The model under review builds one solid part; all positions refer to its coordinate system, in mm. Coordinates: 2 decimals unless noted, no trailing zeros. Write each loop counter-clockwise with the first axis right and the second up, starting at its lowest first coordinate (ties: lowest second). Pieces come first, ordered by that corner, then holes. Notation, with made-up numbers: (-5.5, -8) - (46.5, -8) arc R27 ccw to (46.5, 17) - close; hole circle Ø9 at (28, 17). An arc over 180 degrees is marked (long way). Answer as CSV lines item,"result". Start each with the question number.
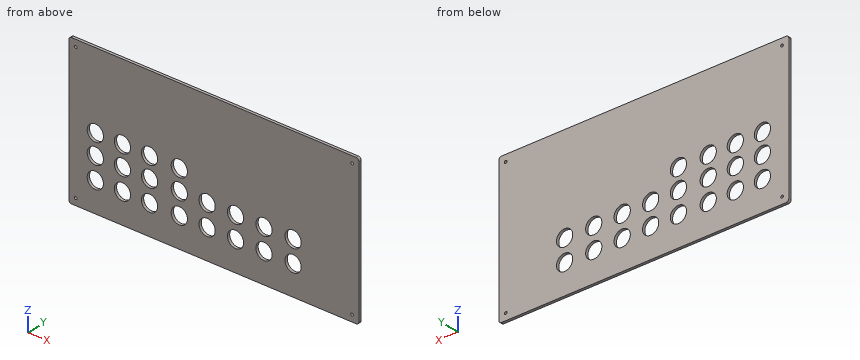
```python
from build123d import *

# Parameters (mm, degrees)
BOSS_EXTRUDE1_DEPTH       = 2
SKETCH3_R                 = 6
CUT_EXTRUDE1_DEPTH        = 3
F_2_0MM_DOWEL_HOLE1_D     = 2
F_2_0MM_DOWEL_HOLE1_DEPTH = 8
F_2_0MM_DOWEL_HOLE1_TIP   = 0.600860619


with BuildPart() as part:
    # Sketch2 → Boss-Extrude1 (new body)
    with BuildSketch(Plane(origin=(0, 0, 0), x_dir=(1, 0, 0), z_dir=(0, 1, 0))):
        with BuildLine():
            Line((105, 54.5), (-105, 54.5))
            ThreePointArc((-105, 54.5), (-106.414213562, 53.914213562), (-107, 52.5))
            Line((-107, 52.5), (-107, -52.5))
            ThreePointArc((-107, -52.5), (-106.414213562, -53.914213562), (-105, -54.5))
            Line((-105, -54.5), (105, -54.5))
            ThreePointArc((105, -54.5), (106.414213562, -53.914213562), (107, -52.5))
            Line((107, -52.5), (107, 52.5))
            ThreePointArc((107, 52.5), (106.414213562, 53.914213562), (105, 54.5))
        make_face()
    extrude(amount=BOSS_EXTRUDE1_DEPTH)

    # Sketch3 → Cut-Extrude1 (cut)
    with BuildSketch(Plane(origin=(0, 2, 0), x_dir=(1, 0, 0), z_dir=(0, 1, 0))):
        with Locations((-87.5, 32.5)):
            Circle(SKETCH3_R)
        with Locations((-67.5, 32.5)):
            Circle(SKETCH3_R)
        with Locations((-47.5, 32.5)):
            Circle(SKETCH3_R)
        with Locations((-25.5, 32.5)):
            Circle(SKETCH3_R)
        with Locations((-5, 32.5)):
            Circle(SKETCH3_R)
        with Locations((16, 32.5)):
            Circle(SKETCH3_R)
        with Locations((37, 32.5)):
            Circle(SKETCH3_R)
        with Locations((58.5, 32.5)):
            Circle(SKETCH3_R)
        with Locations((-87.5, 16.5)):
            Circle(SKETCH3_R)
        with Locations((-67.5, 16.5)):
            Circle(SKETCH3_R)
        with Locations((-47.5, 16.5)):
            Circle(SKETCH3_R)
        with Locations((-25.5, 16.5)):
            Circle(SKETCH3_R)
        with Locations((-5, 16.5)):
            Circle(SKETCH3_R)
        with Locations((16, 16.5)):
            Circle(SKETCH3_R)
        with Locations((37, 16.5)):
            Circle(SKETCH3_R)
        with Locations((58.5, 16.5)):
            Circle(SKETCH3_R)
        with Locations((-67.5, 1.5)):
            Circle(SKETCH3_R)
        with Locations((-87.5, 1.5)):
            Circle(SKETCH3_R)
        with Locations((-47.5, 1.5)):
            Circle(SKETCH3_R)
        with Locations((-25.5, 1.5)):
            Circle(SKETCH3_R)
    extrude(amount=-CUT_EXTRUDE1_DEPTH, mode=Mode.SUBTRACT)

    # Ø2.0mm Dowel Hole1
    with Locations(Plane(origin=(0, 2, 0), x_dir=(1, 0, 0), z_dir=(0, 1, 0))):
        with Locations((-102, 49.5), (102, 49.5), (102, -49.5), (-102, -49.5)):
            Hole(F_2_0MM_DOWEL_HOLE1_D / 2, depth=F_2_0MM_DOWEL_HOLE1_DEPTH)
            with Locations((0, 0, -(F_2_0MM_DOWEL_HOLE1_DEPTH + F_2_0MM_DOWEL_HOLE1_TIP / 2))):  # 118° drill point
                Cone(0, F_2_0MM_DOWEL_HOLE1_D / 2, F_2_0MM_DOWEL_HOLE1_TIP, mode=Mode.SUBTRACT)


solid = part.part
```
(1) Add section B-B on y = 0.6. Give the number of separate pieces and of enclosed holes in the cut face, then the cut area to 3 significant figures.
(2) For pin 1 (11 mm diameter, centred on x = -25.5, z = -16.5, fed in from +Y) (3 decimals), flat-tipped, find the tip position at first contact; note if it passes through.
(3) Add section C-C on x = 16. Give the boundary of the cut face in (y, z).
(4) Wall thickness on line 1 (Z direction, x = -25.5, y = 0.6); line 2 (Z direction, x = -69, y = 0.55); line 3 (X direction, y = 0.7, z = -2.5): over which ranges is each line inside the solid? List them lowest first.
(5) Add section A-A on x = -67.5. Give the boundary of the cut face in (y, z), then the cut area to 3 significant figures.
Reported:
1,separate pieces,"1"
1,enclosed holes,"24"
1,area,"21,000 mm²"
2,pin 1,"through"
3,outline,"(0, -54.5) - (2, -54.5) - (2, -38.5) - (0, -38.5) - close; (0, -26.5) - (2, -26.5) - (2, -22.5) - (0, -22.5) - close; (0, -10.5) - (2, -10.5) - (2, 54.5) - (0, 54.5) - close"
4,line 1,"-54.5 to -38.5, -26.5 to -22.5, -10.5 to -7.5, 4.5 to 54.5"
4,line 2,"-54.5 to -38.31, -26.69 to -22.31, -10.69 to -7.31, 4.31 to 54.5"
4,line 3,"-107 to -93.42, -81.58 to -73.42, -61.58 to -53.42, -41.58 to -31.42, -19.58 to 107"
5,outline,"(0, -54.5) - (2, -54.5) - (2, -38.5) - (0, -38.5) - close; (0, -26.5) - (2, -26.5) - (2, -22.5) - (0, -22.5) - close; (0, -10.5) - (2, -10.5) - (2, -7.5) - (0, -7.5) - close; (0, 4.5) - (2, 4.5) - (2, 54.5) - (0, 54.5) - close"
5,area,"146 mm²"
